Here's how the part is built. I have some questions about the finished solid (model axes, mm). Face numbers are marked on the shaded views. A direction names the side the tool comes from. Coordinates: 2 decimals unless noted, no trailing zeros. Write each loop counter-clockwise with the first axis right and the second up, starting at its lowest first coordinate (ties: lowest second). Pieces come first, ordered by that corner, then holes. Notation, with made-up numbers: (23, -32) - (36, -32) arc R18 cw to (36, -3) - close; hole circle Ø10 at (-28.75, 86). An arc over 180 degrees is marked (long way). Answer in a Markdown table with one row per item. Add a question column.
Item 1: If I drill on probe 1 along X at (y, z) = (0, -3); probe 2 along Y at (x, z) = (126, 0.25); probe 3 along X at (y, z) = (-6.25, 3.25), over which ranges is the centre line in solid material (lowest first)? Write a range as from..to.
Item 2: Imagine slicing it at D-D (x = 80.5). Please give me the cut outline in (y, z), plus the area to 3 significant figures.
Item 3: Imagine slicing it at C-C (x = 126). Please give me the cut outline in (y, z), plus the area to 3 significant figures.
Item 4: Imagine slicing it at A-A (y = 0). Please give me the cut outline in (x, z), plus the area to 3 significant figures.
Item 5: I'm going to push flat-ended pins straight in: pin 1 (8 mm diameter, centred on x = 118, z = 5.5, fed in from +Y); pin 2 (4 mm diameter, centred on x = 87, y = -1, fed in from -Z); pin 3 (6 mm diameter, centred on x = 87, y = -5.5, fed in from +Z). Where does each tip first touch, or does it pass through?
Item 6: Which directions (+Z, -Z, +X, -X, +Y, -Y) give clear straight access to the entire face, cutting with the end or side of a thin tool? Please do the marked faces 1 and 2.
Item 7: Imagine slicing it at B-B (z = 0). Please give me the cut outline in (x, y).
Item 8: We'd pull the mould along X, two halves only. Please class the marked faces 3, 4 and 5: +X half, -X half, draft (parallel to the pull), parting line (faces both ways), or undercut.
Autodesk Inventor part; units mm, degrees
ref_plane "YZ Plane" through (0, 0, 0) normal (1, 0, 0) x (0, 1, 0)
ref_plane "XZ Plane" through (0, 0, 0) normal (0, 1, 0) x (-1, 0, 0)
ref_plane "XY Plane" through (0, 0, 0) normal (0, 0, 1) x (1, 0, 0)
sketch "Esboço1" plane through (0, 0, 0) normal (0, 0, 1) x (1, 0, 0)
  line L0 (0, 0) -> (0, 6)
  line L1 (0, 6) -> (4, 6)
  line L2 (4, 6) -> (4, 4)
  line L3 (4, 4) -> (8, 4)
  line L4 (8, 4) -> (8, 6)
  line L5 (8, 6) -> (16, 6)
  line L6 (16, 6) -> (16, 8)
  line L7 (16, 8) -> (104, 8)
  line L8 (104, 8) -> (104, 6)
  line L9 (104, 6) -> (114, 6)
  line L10 (114, 6) -> (114, 9)
  line L11 (114, 9) -> (138, 9)
  line L12 (138, 9) -> (138, 0)
  line L13 (138, 0) -> (0, 0)
  dimension "d0" = 6
  dimension "d1" = 4
  dimension "d2" = 2
  dimension "d3" = 4
  dimension "d4" = 2
  dimension "d5" = 8
  dimension "d6" = 2
  dimension "d7" = 88
  dimension "d11" = 2
  dimension "d12" = 10
  dimension "d13" = 3
  dimension "d14" = 24
revolve "Revolução1" add sketch "Esboço1" angle 360 about axis through (138, 0, 0) along (-1, 0, 0)
sketch "Esboço2" plane through (0, 0, 0) normal (0, 0, 1) x (1, 0, 0)
  line L0 (138, -9) -> (138, 9)
  line L1 (138, 0) -> (126, 0)
  point P0 (0, 0)
  dimension "d16" = 12
hole "Furo1" at (126, 0, 0) direction (0, 0, -1) diameter 6 end through all both
thread "Rosca1"
properties part number "haste_roscada" material "Aluminum 6061-AHC"
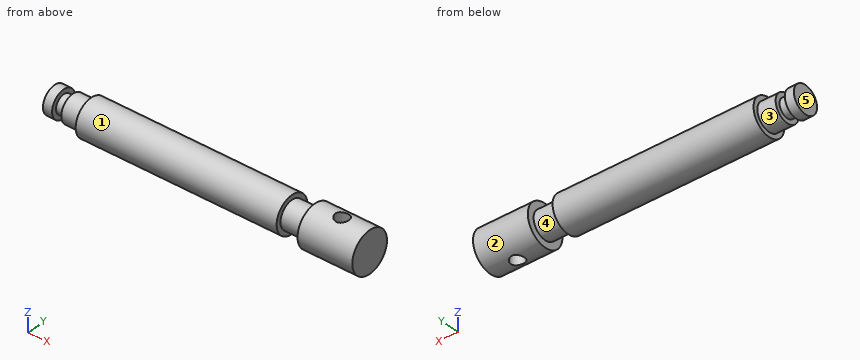
Here are the results:
| question | item | result |
|---|---|---|
| 1 | probe 1 | x = 0..123, 129..138 |
| 1 | probe 2 | y = -9..-3, 3..9 |
| 1 | probe 3 | x = 16..104, 114..138 |
| 2 | outline | circle Ø16 at (0, 0) |
| 2 | area | 201 mm2 |
| 3 | outline | (-3, -8.49) - (-3, 8.49) arc R9 ccw to start; (3, -8.49) arc R9 ccw to (3, 8.49) - close |
| 3 | area | 149 mm2 |
| 4 | outline | (0, -6) - (4, -6) - (4, -4) - (8, -4) - (8, -6) - (16, -6) - (16, -8) - (104, -8) - (104, -6) - (114, -6) - (114, -9) - (123, -9) - (123, 9) - (114, 9) - (114, 6) - (104, 6) - (104, 8) - (16, 8) - (16, 6) - (8, 6) - (8, 4) - (4, 4) - (4, 6) - (0, 6) - close; (129, -9) - (138, -9) - (138, 9) - (129, 9) - close |
| 4 | area | 2,030 mm2 |
| 5 | pin 1 | stops at y = 8.87 |
| 5 | pin 2 | stops at z = -8 |
| 5 | pin 3 | stops at z = 7.6 |
| 6 | face 1 | -X |
| 6 | face 2 | +X, -X |
| 7 | outline | (0, -6) - (4, -6) - (4, -4) - (8, -4) - (8, -6) - (16, -6) - (16, -8) - (104, -8) - (104, -6) - (114, -6) - (114, -9) - (138, -9) - (138, 9) - (114, 9) - (114, 6) - (104, 6) - (104, 8) - (16, 8) - (16, 6) - (8, 6) - (8, 4) - (4, 4) - (4, 6) - (0, 6) - close; hole circle Ø6 at (126, 0) |
| 8 | face 3 | draft |
| 8 | face 4 | undercut |
| 8 | face 5 | -X half |
